from build123d import *

# Parameters (mm, degrees)
F1_DEPTH = 15


with BuildPart() as f1:
    # F0 (on Front) → F1 (new body)
    with BuildSketch(Plane.XZ):
        with BuildLine():
            ThreePointArc((-31.990636, 2.988535), (-31.980754, 0.994284), (-30.252016, 0))
            Line((-30.252016, 0), (0, 0))
            Line((0, 0), (4.023837, 3.83522))
            ThreePointArc((4.023837, 3.83522), (4.639042, 5.142749), (4.212761, 6.52347))
            Line((4.212761, 6.52347), (-0.127799, 12.012706))
            Line((-0.127799, 12.012706), (-13.884482, 12.012706))
            Line((-13.884482, 12.012706), (-23.950903, 12.012706))
            ThreePointArc((-23.950903, 12.012706), (-26.465193, 11.334552), (-28.297452, 9.484045))
            Line((-28.297452, 9.484045), (-31.990636, 2.988535))
        make_face()
    extrude(amount=F1_DEPTH)


solid = f1.part
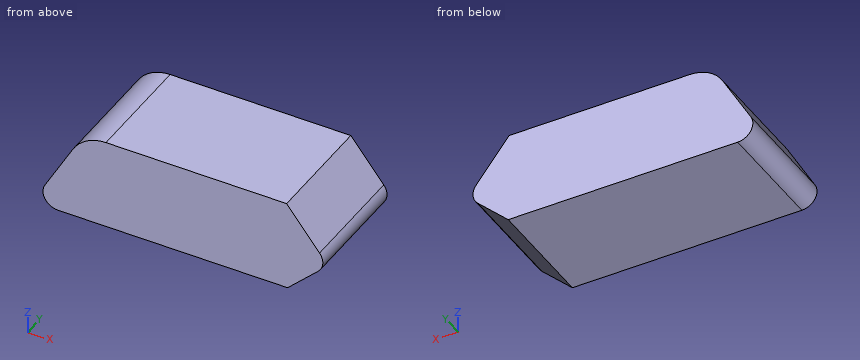
Geometry check sheet. Reference: the model listing, model coordinates, mm. Give positions to 0.01 mm unless a question says otherwise; leave off trailing zeros. Order: outer loops, then holes, each group sorted by start corner. A loop starts at its lowest first (then second) coordinate and runs counter-clockwise, first axis right, second up. Notation, with made-up numbers: M 13,75.5 L 69,75.5 A20 ccw 69,91.5 Z; hole C 21,37 d11. An arc over 180 degrees is marked long. Use a Markdown table: item, result.
Item 1: Section check A-A (y = -6.25). Record the cut outline in (x, z).
Answers follow:
| item | result |
|---|---|
| outline | M -31.99,2.99 A2 ccw -30.25,0 L 0,0 L 4.02,3.84 A2 ccw 4.21,6.52 L -0.13,12.01 L -23.95,12.01 A5 ccw -28.3,9.48 Z |
Item 2: Material ranges on line 1 along Z through (x, y) = (0, -9); line 2 along X through (y, z) = (-14, 5.75); line 3 along X through (y, z) = (-12.5, 3.5), recorded low to high.
Answers follow:
| item | result |
|---|---|
| line 1 | z = 0 to 11.85 |
| line 2 | x = -30.42 to 4.59 |
| line 3 | x = -31.7 to 3.67 |
Item 3: Section check C-C (x = -27). Record the cut outline in (y, z).
Answers follow:
| item | result |
|---|---|
| outline | M -15,0 L 0,0 L 0,10.98 L -15,10.98 Z |
Item 4: Depth check by flat-ended pin: P1, Ø2, axis at y = -4.5, z = 8, coming from the +X side. Enter the tip coordinate at first touch or a pass-through.
Answers follow:
| item | result |
|---|---|
| P1 | stops at x = 3.84 |
Item 5: Section check B-B (z = 1.75). Record the cut outline in (x, y).
Answers follow:
| item | result |
|---|---|
| outline | M -32.24,-15 L 1.84,-15 L 1.84,0 L -32.24,0 Z |
